Source: CAD feature listing. Evaluate the final solid. Frame: model axes, mm. A direction names the side the tool comes from. Round coordinates to 2 decimals unless told otherwise and drop trailing zeros. Order: outer loops, then holes, each group sorted by start corner. A loop starts at its lowest first (then second) coordinate and runs counter-clockwise, first axis right, second up. Notation, with made-up numbers: (71, -18) -> (75, -18) arc R35 ccw to (75, 14) -> close; hole circle Ø6 at (29.25, 63.25). An arc over 180 degrees is marked (long way). Answer as CSV lines item,"result". Start each with the question number.
(1) Pull-direction query (X, two-part tool) for faces 5 (the flat face through (53, 15, 14)), 6 (the flat face through (26, 53, 2)), 7 (the flat face through (3, 16, 9)), 8 (the cylindrical face through (26.192, 16.504, 1.972)); classes: +X half, -X half, draft (parallel to the pull), parting line (faces both ways), or undercut.
(2) Section query C-C (y = 46). Output: boundary loops of the cut face in (x, z), plus the area to 3 significant figures.
(3) Section query A-A (z = 30). Output: boundary loops of the cut face in (x, y), plus the area to 3 significant figures.
(4) Contact query for flat-ended pins moving along their axis: P1, Ø21, axis at x = 25.5, z = 46.5, coming from the +Y side; P2, Ø5, axis at x = 26.5, z = 30, coming from the +Y side; P3, Ø6.5, axis at x = 44.1, y = 28.5, coming from the +Z side; P4, Ø8, axis at x = 22.5, y = 40, coming from the +Z side. Output: stop coordinate, or through.
(5) Section query B-B (x = 44.1). Output: boundary loops of the cut face in (y, z).
(6) Line query: line 1 along Z through (x, y) = (26.5, 0.95); line 2 along Y through (x, z) = (44.1, 1.75); line 3 along X through (y, z) = (28, 2). Output: solid intervals per line, ascending. Write a range as from..to.
(7) Section query D-D (y = 28.5). Output: boundary loops of the cut face in (x, z), plus the area to 3 significant figures.
(8) Set-up query: faces 1 (the flat face through (20, 0, 30)), 2 (the flat face through (14, 6, 36)), 3 (the flat face through (15.674, 5, 37)), 4 (the cylindrical face through (26.7, 46.9, 2)). Return all of +Z, -Z, +X, -X, +Y, -Y with unobstructed straight access to the full face (end or side cutting, diameter ignored); none if empty.
```python
from build123d import *

# Parameters (mm, degrees)
ESBO_O1_W                  = 53
ESBO_O1_H                  = 53
RESSALTO_EXTRUS_O1_DEPTH   = 4
ESBO_O2_W                  = 53
ESBO_O2_H                  = 4
RESSALTO_EXTRUS_O2_DEPTH   = 60
CORTE_EXTRUS_O1_DEPTH      = 21
CORTE_EXTRUS_O1_DEPTH_BACK = 18
CORTE_EXTRUS_O2_DEPTH      = 17
CORTE_EXTRUS_O2_DEPTH_BACK = 15
ESBO_O4_R                  = 2
ESBO_O5_W                  = 3
ESBO_O5_H                  = 36.373853852
RESSALTO_EXTRUS_O3_DEPTH   = 17
CORTE_EXTRUS_O3_DEPTH      = 53
ESBO_O7_W                  = 26.228570329
ESBO_O7_H                  = 46.898944641
ESBO_O7_W_2                = 20
ESBO_O7_H_2                = 41
RESSALTO_EXTRUS_O4_DEPTH   = 6
CORTE_EXTRUS_O4_DEPTH      = 10
CORTE_EXTRUS_O4_DEPTH_BACK = 21
ESBO_O8_R                  = 2


# Read off the part's stored shape, not the designer's step: Corte-extrus_o3
with BuildPart() as part:
    # Esbo_o1 → Ressalto-extrus_o1 (new body)
    with BuildSketch(Plane.XY):
        with Locations((26.5, 26.5)):
            Rectangle(ESBO_O1_W, ESBO_O1_H)
    extrude(amount=RESSALTO_EXTRUS_O1_DEPTH)

    # Esbo_o2 → Ressalto-extrus_o2 (add)
    with BuildSketch(Plane.XY):
        with Locations((26.5, 2)):
            Rectangle(ESBO_O2_W, ESBO_O2_H)
    extrude(amount=RESSALTO_EXTRUS_O2_DEPTH)

    # Esbo_o3 → Corte-extrus_o1 (cut, two sides: drawn at the far end of the back side and taken through both)
    with BuildSketch(Plane.XY.offset(-CORTE_EXTRUS_O1_DEPTH_BACK)):
        with BuildLine():
            Line((17.098198891, 39.704586726), (14.91581435, 31.631555975))
            ThreePointArc((14.91581435, 31.631555975), (26.5, 16.5), (38.08418565, 31.631555975))
            Line((38.08418565, 31.631555975), (35.901801109, 39.704586726))
            ThreePointArc((35.901801109, 39.704586726), (26.5, 46.902274107), (17.098198891, 39.704586726))
        make_face()
    extrude(amount=CORTE_EXTRUS_O1_DEPTH + CORTE_EXTRUS_O1_DEPTH_BACK, mode=Mode.SUBTRACT)

    # Esbo_o4 → Corte-extrus_o2 (cut, two sides: drawn at the far end of the back side and taken through both)
    with BuildSketch(Plane.XY.offset(-CORTE_EXTRUS_O2_DEPTH_BACK)):
        with Locations(Location((8.9, 28.5, 0), (0, 0, 180))):
            Circle(ESBO_O4_R)
        with Locations(Location((44.1, 28.5, 0), (0, 0, 180))):
            Circle(ESBO_O4_R)
    extrude(amount=CORTE_EXTRUS_O2_DEPTH + CORTE_EXTRUS_O2_DEPTH_BACK, mode=Mode.SUBTRACT)

    # Esbo_o5 → Ressalto-extrus_o3 (add)
    with BuildSketch(Plane.XY):
        with Locations((1.5, 18.186926926)):
            Rectangle(ESBO_O5_W, ESBO_O5_H)
        with Locations((51.5, 18.186926926)):
            Rectangle(ESBO_O5_W, ESBO_O5_H)
    extrude(amount=RESSALTO_EXTRUS_O3_DEPTH)

    # Corte-extrus_o3 outline → Corte-extrus_o3 (cut)
    with BuildSketch(Plane(origin=(0, 0, 0), x_dir=(0, 0, -1), z_dir=(1, 0, 0))):
        with BuildLine():
            ThreePointArc((-17, 5.226597996), (-13.510052949, 22.056538471), (-4, 36.373853852))
            Line((-4, 36.373853852), (-17, 36.373853852))
            Line((-17, 36.373853852), (-17, 5.226597996))
        make_face()
    extrude(amount=CORTE_EXTRUS_O3_DEPTH, mode=Mode.SUBTRACT)

    # Esbo_o7 → Ressalto-extrus_o4 (add)
    with BuildSketch(Plane(origin=(0, 0, 0), x_dir=(1, 0, 0), z_dir=(0, 1, 0))):
        with Locations((25.531831297, -36.55052768)):
            Rectangle(ESBO_O7_W, ESBO_O7_H)
        with Locations((25.674113589, -36.5)):
            Rectangle(ESBO_O7_W_2, ESBO_O7_H_2, mode=Mode.SUBTRACT)
    extrude(amount=RESSALTO_EXTRUS_O4_DEPTH)

    # Esbo_o8 → Corte-extrus_o4 (cut, two sides: drawn at the far end of the back side and taken through both)
    with BuildSketch(Plane(origin=(0, 0, 0), x_dir=(1, 0, 0), z_dir=(0, 1, 0)).offset(-CORTE_EXTRUS_O4_DEPTH_BACK)):
        with Locations(Location((26.5, -30, 0), (0, 0, 270))):
            Circle(ESBO_O8_R)
    extrude(amount=CORTE_EXTRUS_O4_DEPTH + CORTE_EXTRUS_O4_DEPTH_BACK, mode=Mode.SUBTRACT)


solid = part.part
```
Answer block:
1,face 5,"+X half"
1,face 6,"draft"
1,face 7,"undercut"
1,face 8,"undercut"
2,outline,"(0, 0) -> (22.41, 0) -> (22.41, 4) -> (0, 4) -> close; (30.59, 0) -> (53, 0) -> (53, 4) -> (30.59, 4) -> close"
2,area,"179 mm2"
3,outline,"(0, 0) -> (24.5, 0) -> (24.5, 4) -> (15.67, 4) -> (15.67, 6) -> (12.42, 6) -> (12.42, 4) -> (0, 4) -> close; (28.5, 0) -> (53, 0) -> (53, 4) -> (38.65, 4) -> (38.65, 6) -> (35.67, 6) -> (35.67, 4) -> (28.5, 4) -> close"
3,area,"208 mm2"
4,P1,"y = 6"
4,P2,"y = 4"
4,P3,"z = 4"
4,P4,"through"
5,outline,"(0, 0) -> (26.5, 0) -> (26.5, 4) -> (4, 4) -> (4, 60) -> (0, 60) -> close; (30.5, 0) -> (53, 0) -> (53, 4) -> (30.5, 4) -> close"
6,line 1,"0..28, 32..60"
6,line 2,"0..26.5, 30.5..53"
6,line 3,"0..6.96, 10.84..14.51, 38.49..42.16, 46.04..53"
7,outline,"(0, 0) -> (6.9, 0) -> (6.9, 4) -> (3, 4) -> (3, 10.19) -> (0, 10.19) -> close; (10.9, 0) -> (14.5, 0) -> (14.5, 4) -> (10.9, 4) -> close; (38.5, 0) -> (42.1, 0) -> (42.1, 4) -> (38.5, 4) -> close; (46.1, 0) -> (53, 0) -> (53, 10.19) -> (50, 10.19) -> (50, 4) -> (46.1, 4) -> close"
7,area,"121 mm2"
8,face 1,"+Z, -Z, +X, -X, -Y"
8,face 2,"+Z, +Y"
8,face 3,"+Y"
8,face 4,"+Z, -Z"
